```python
from build123d import *

# Parameters (mm, degrees)
SKETCH1_R           = 9
BOSS_EXTRUDE1_DEPTH = 64.5
FILLET1_R           = 0.5
SKETCH2_R           = 2.962162188
BOSS_EXTRUDE2_DEPTH = 0.5
FILLET2_R           = 0.2


with BuildPart() as part:
    # Sketch1 → Boss-Extrude1 (new body)
    with BuildSketch(Plane.XY):
        Circle(SKETCH1_R)
    extrude(amount=BOSS_EXTRUDE1_DEPTH)

    # Fillet1
    fillet1_edges = [part.edges().sort_by_distance(p)[0] for p in [
        (-9, 0, 0),
        (-9, 0, 64.5),
    ]]
    fillet(fillet1_edges, radius=FILLET1_R)

    # Sketch2 → Boss-Extrude2 (add)
    with BuildSketch(Plane.XY.offset(64.5)):
        Circle(SKETCH2_R)
    extrude(amount=BOSS_EXTRUDE2_DEPTH)

    # Fillet2
    fillet2_edges = [part.edges().sort_by_distance(p)[0] for p in [
        (-2.962162188, 0, 65),
    ]]
    fillet(fillet2_edges, radius=FILLET2_R)


solid = part.part
```
Check sheet for the modelled part. Datum: model origin and axes. Units: mm. Coordinates: 2 decimals unless noted, no trailing zeros. Loops run counter-clockwise (first coordinate to the right, second up) from the corner with the lowest first, then second, coordinate; pieces in that order, holes last. Notation, with made-up numbers: M 78.25,-20 L 127.25,-20 A17 cw 127.25,-6 Z; hole C 45.25,-28.5 d8. An arc over 180 degrees is marked long. Answer as a JSON object with one key per item and string values.
1. Release check for a two-part mould opening along Y. For faces 1 (the flat face through (4, 0, 64.5)), 2 (the cylindrical face through (1.59, 2.5, 64.65)) record: pulls with the +Y half, pulls with the -Y half, needs draft (parallel to the pull), parting line crosses it, or undercut.
Outcome:
{"face 1": "needs draft", "face 2": "parting line crosses it"}
2. Sectioned sample at A-A on z = 9. Record the cut outline in (x, y).
Outcome:
{"outline": "C 0,0 d18"}
3. Depth check by flat-ended pin: P1, Ø1.5, axis at y = 4, z = 29, coming from the +X side; P2, Ø6, axis at y = -4.5, z = 54.5, coming from the +X side; P3, Ø2, axis at x = -5.5, z = 15.5, coming from the -Y side. Enter the tip coordinate at first touch or a pass-through.
Outcome:
{"P1": "x = 8.39", "P2": "x = 8.87", "P3": "y = -7.79"}
4. Scan lines: L1, parallel to Z at x = -6.5, y = -4.5; L2, parallel to Y at x = -0.5, z = 35.5; L3, parallel to Y at x = -7.25, z = 37. Record each from-to range of solid material in increasing order. Write a range as from..to.
Outcome:
{"L1": "0..64.5", "L2": "-8.99..8.99", "L3": "-5.33..5.33"}
